```python
from build123d import *

# Parameters (mm, degrees)
ESQUISSE1_W             = 150
ESQUISSE1_H             = 100
BOSS_EXTRU_1_DEPTH      = 75
ENL_V_MAT_EXTRU_2_DEPTH = 70
ESQUISSE5_R             = 4
ENL_V_MAT_EXTRU_3_DEPTH = 3
ESQUISSE6_R             = 4
ENL_V_MAT_EXTRU_4_DEPTH = 3


with BuildPart() as part:
    # Esquisse1 → Boss.-Extru.1 (new body)
    with BuildSketch(Plane.XY):
        with Locations((23.806447762, -50)):
            Rectangle(ESQUISSE1_W, ESQUISSE1_H)
    extrude(amount=BOSS_EXTRU_1_DEPTH)

    # Esquisse2 → Enlèv. mat.-Extru.2 (cut)
    with BuildSketch(Plane.XY.offset(75)):
        Polygon((-37.193552238, -4), (84.806447762, -4), (94.806447762, -14), (94.806447762, -86), (84.806447762, -96), (-37.193552238, -96), (-47.193552238, -86), (-47.193552238, -14), align=None)
    extrude(amount=-ENL_V_MAT_EXTRU_2_DEPTH, mode=Mode.SUBTRACT)

    # Esquisse5 → Enlèv. mat.-Extru.3 (cut)
    with BuildSketch(Plane.XY.offset(75)):
        with Locations((-45.7114952, -5.446962242)):
            Circle(ESQUISSE5_R)
    extrude(amount=-ENL_V_MAT_EXTRU_3_DEPTH, mode=Mode.SUBTRACT)

    # Esquisse6 → Enlèv. mat.-Extru.4 (cut)
    with BuildSketch(Plane.XY.offset(75)):
        with Locations((92.954779507, -5.115671586)):
            Circle(ESQUISSE6_R)
        with Locations((92.526014057, -95.195707231)):
            Circle(ESQUISSE6_R)
        with Locations((-45.931001662, -94.321365955)):
            Circle(ESQUISSE6_R)
    extrude(amount=-ENL_V_MAT_EXTRU_4_DEPTH, mode=Mode.SUBTRACT)


solid = part.part
```
Work out the finished part from the listing and answer in its coordinate system (mm). A direction names the side the tool comes from. Give positions to 0.01 mm unless a question says otherwise; leave off trailing zeros. Order: outer loops, then holes, each group sorted by start corner. A loop starts at its lowest first (then second) coordinate and runs counter-clockwise, first axis right, second up. Notation, with made-up numbers: (2, -7.5) -> (51, -7.5) arc R16 cw to (51, 1.5) -> close; hole circle Ø5 at (70.5, -32). An arc over 180 degrees is marked (long way). Answer as CSV lines item,"result". Start each with the question number.
(1) Section A-A, the plane y = -20.5 is taken. Write down the section's boundary in (x, z), plus the area to 3 significant figures.
(2) Consider line 1 along Y through (x, z) = (62.5, 16.5); line 2 along X through (y, z) = (-21, 43); line 3 along Z through (x, y) = (-15.5, -65.5). Determine where each line is inside the solid, lowest interval first.
(3) Each of these flat-tipped pins is pushed along its axis until it touches: pin 1 Ø5 at (x, y) = (-30.5, -84.5) entering from +Z; pin 2 Ø4 at (x, y) = (92.5, -3.5) entering from +Z. Where does it stop, or does it pass through?
(4) Section B-B, the plane z = 14 is taken. Write down the section's boundary in (x, y), plus the area to 3 significant figures.
(5) Section C-C, the plane x = 9 is taken. Write down the section's boundary in (y, z).
(6) For a pull along Y with two mould halves and no side action, classify faces 3 (the flat face through (23, -2, 75)), 4 (the flat face through (25, -49, 5)), 5 (the flat face through (23, 0, 37)) as released by +Y, released by -Y, zero draft, split by the parting line, or undercut.
(7) Which of the six approach directions +Z, -Z, +X, -X, +Y, -Y give full straight-line access (tool end or side, diameter ignored) to faces 1 (the flat face through (98.806, -51, 37)), 2 (the cylindrical face through (-41.896, -4.245, 73.521))?
Entries:
1,outline,"(-51.19, 0) -> (98.81, 0) -> (98.81, 75) -> (94.81, 75) -> (94.81, 5) -> (-47.19, 5) -> (-47.19, 75) -> (-51.19, 75) -> close"
1,area,"1,310 mm²"
2,line 1,"-100 to -96, -4 to 0"
2,line 2,"-51.19 to -47.19, 94.81 to 98.81"
2,line 3,"0 to 5"
3,pin 1,"z = 5"
3,pin 2,"z = 72"
4,outline,"(-51.19, -100) -> (98.81, -100) -> (98.81, 0) -> (-51.19, 0) -> close; hole (-47.19, -86) -> (-37.19, -96) -> (84.81, -96) -> (94.81, -86) -> (94.81, -14) -> (84.81, -4) -> (-37.19, -4) -> (-47.19, -14) -> close"
4,area,"2,140 mm²"
5,outline,"(-100, 0) -> (0, 0) -> (0, 75) -> (-4, 75) -> (-4, 5) -> (-96, 5) -> (-96, 75) -> (-100, 75) -> close"
6,face 3,"zero draft"
6,face 4,"undercut"
6,face 5,"released by +Y"
7,face 1,"+Z, -Z, +X, +Y, -Y"
7,face 2,"+Z"
